The drawing under review shows one solid part. Ordinate dimensions are in mm from its lowest x, y, z. A direction names the side the tool comes from. Round coordinates to 2 decimals unless told otherwise and drop trailing zeros. Order: outer loops, then holes, each group sorted by start corner. A loop starts at its lowest first (then second) coordinate and runs counter-clockwise, first axis right, second up. Notation, with made-up numbers: (69.25, 12) -> (119.25, 12) arc R30 ccw to (119.25, 36) -> close; hole circle Ø8 at (-35, 55). An arc over 180 degrees is marked (long way). Use a Markdown table: item, result. Add a question column.
1) Consider section B-B (z = 4). State the section outline as (x, y) points (3 decimals).
2) Consider section D-D (x = 2.5). State the section outline as (y, z) points, plus the area to 3 significant figures.
3) Machinability: for the marked faces 1 and 2, which of the approach directions +Z, -Z, +X, -X, +Y, -Y give a long, thin tool a straight path to every point of the face, cutting with its end or side? Answer none if there is none.
4) Consider section C-C (x = 7). State the section outline as (y, z) points, plus the area to 3 significant figures.
5) Clearance check with flat-ended pins moving along their axes: P1, Ø6, axis at y = 13, z = 7, coming from the -X side; P2, Ø6, axis at x = 9.5, z = 12, coming from the -Y side (3 decimals); P3, Ø3, axis at x = 2, z = 12.5, coming from the +Y side; P4, Ø4, axis at x = 8, z = 15, coming from the +Y side (3 decimals). State where each tip first meets the part, or that it passes through.
6) Consider section A-A (y = 13.5). State the section outline as (x, z) points (3 decimals).
7) Draft analysis for pull direction Z (two halves, no side actions). For the marked faces 3, 4 and 5, state which applies: pulls with the +Z half, pulls with the -Z half, needs draft (parallel to the pull), parting line crosses it, or undercut.
8) Wall thickness on line 1 along X through (y, z) = (4.25, 4) (3 decimals); line 2 along Z through (x, y) = (11, 13.5); line 3 along X through (y, z) = (0.5, 4.75): over which ranges is each line inside the solid? List them lowest first. Write a range as [from, to].
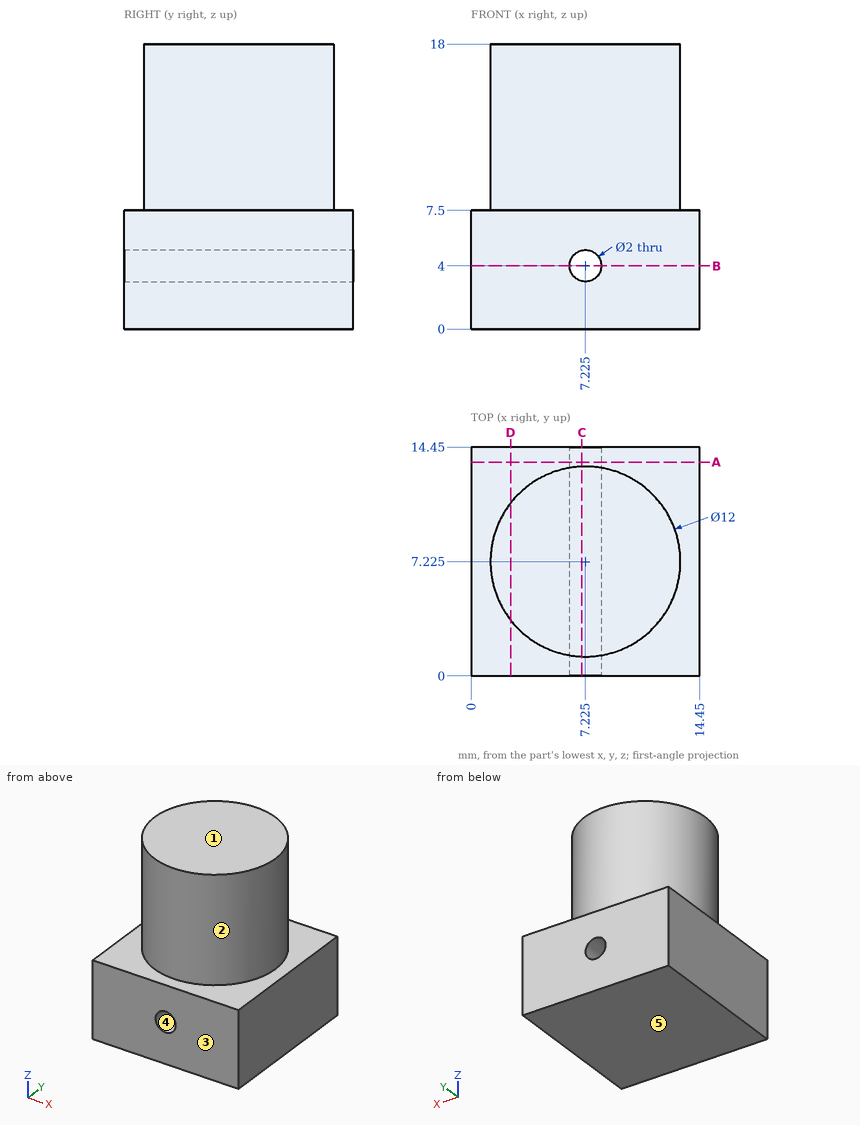
Results list:
| question | item | result |
|---|---|---|
| 1 | outline | (0, 0) -> (6.225, 0) -> (6.225, 14.45) -> (0, 14.45) -> close; (8.225, 0) -> (14.45, 0) -> (14.45, 14.45) -> (8.225, 14.45) -> close |
| 2 | outline | (0, 0) -> (14.45, 0) -> (14.45, 7.5) -> (10.92, 7.5) -> (10.92, 18) -> (3.53, 18) -> (3.53, 7.5) -> (0, 7.5) -> close |
| 2 | area | 186 mm2 |
| 3 | face 1 | +Z, +X, -X, +Y, -Y |
| 3 | face 2 | +Z |
| 4 | outline | (0, 0) -> (14.45, 0) -> (14.45, 3.03) -> (0, 3.03) -> close; (0, 4.97) -> (14.45, 4.97) -> (14.45, 7.5) -> (13.22, 7.5) -> (13.22, 18) -> (1.23, 18) -> (1.23, 7.5) -> (0, 7.5) -> close |
| 4 | area | 206 mm2 |
| 5 | P1 | x = 0 |
| 5 | P2 | y = 1.225 |
| 5 | P3 | y = 11.93 |
| 5 | P4 | y = 13.225 |
| 6 | outline | (0, 0) -> (14.45, 0) -> (14.45, 7.5) -> (0, 7.5) -> close; hole circle Ø2 at (7.225, 4) |
| 7 | face 3 | needs draft |
| 7 | face 4 | undercut |
| 7 | face 5 | pulls with the -Z half |
| 8 | line 1 | [0, 6.225], [8.225, 14.45] |
| 8 | line 2 | [0, 7.5] |
| 8 | line 3 | [0, 6.56], [7.89, 14.45] |
